from build123d import *

# Parameters (mm, degrees)
SKETCH1_R                  = 93.345
BASE_DEPTH                 = 4.7625
BASE_DEPTH_BACK            = 4.7625
BOTTOM_SUPPORT_HOLES_DEPTH = 10.525
BOTTOM_SUPPORT_GUIDE_DEPTH = 12.7
SKETCH6_R                  = 1.27
BOTTOM_BOLT_HOLE_DEPTH     = 12.7
TOP_SUPPORT_HOLES_DEPTH    = 4.7625
TOP_SUPPORT_GUIDE_DEPTH    = 12.7
SKETCH12_R                 = 1.27
TOP_BOLT_HOLE_DEPTH        = 12.7
BOTTOM_PATTERN_COUNT       = 4
CIRPATTERN3_COUNT          = 4


with BuildPart() as part:
    # Sketch1 → Base (new body, two sides)
    with BuildSketch(Plane(origin=(0, 0, 0), x_dir=(1, 0, 0), z_dir=(0, 1, 0))) as base_sk:
        Circle(SKETCH1_R)
    extrude(amount=BASE_DEPTH)
    extrude(base_sk.sketch, amount=-BASE_DEPTH_BACK)

    # Sketch2 → Bottom support holes (cut, through all)
    with BuildSketch(Plane(origin=(0, 4.7625, 0), x_dir=(1, 0, 0), z_dir=(0, 1, 0))):
        with BuildLine():
            Line((0, 88.9), (0, 83.82))
            ThreePointArc((0, 83.82), (-21.72026739, 80.956916842), (-41.956713931, 72.563258996))
            Line((-41.956713931, 72.563258996), (-44.39288973, 77.022602796))
            ThreePointArc((-44.39288973, 77.022602796), (-22.977169228, 85.879332172), (0, 88.9))
        make_face()
    bottom_support_holes = extrude(amount=-BOTTOM_SUPPORT_HOLES_DEPTH, mode=Mode.SUBTRACT)

    # Sketch3 → Bottom support guide (add)
    with BuildSketch(Plane(origin=(0, 4.7625, 0), x_dir=(1, 0, 0), z_dir=(0, 1, 0))):
        with BuildLine():
            Line((0, 83.82), (0, 76.2))
            ThreePointArc((0, 76.2), (-19.834896001, 73.573207764), (-38.302281481, 65.8739344))
            Line((-38.302281481, 65.8739344), (-41.956713931, 72.563258996))
            ThreePointArc((-41.956713931, 72.563258996), (-21.72026739, 80.956916842), (0, 83.82))
        make_face()
    bottom_support_guide = extrude(amount=BOTTOM_SUPPORT_GUIDE_DEPTH)

    # Sketch6 → Bottom bolt hole (cut, symmetric)
    with BuildSketch(Plane(origin=(-20.978356966, 0, -78.191629498), x_dir=(-0.965842482, 0, 0.25912989), z_dir=(-0.25912989, 0, -0.965842482))):
        with Locations((-0.00326739, 11.1125)):
            Circle(SKETCH6_R)
    bottom_bolt_hole = extrude(amount=BOTTOM_BOLT_HOLE_DEPTH, both=True, mode=Mode.SUBTRACT)

    # Sketch8 → Top support holes (cut)
    with BuildSketch(Plane(origin=(-31.122978549, 4.7625, 77.296707326), x_dir=(1, 0, 0), z_dir=(0, 1, 0))):
        with BuildLine():
            Line((-31.738814298, 140.158500173), (-28.14671185, 136.566397725))
            ThreePointArc((-28.14671185, 136.566397725), (-41.480754694, 119.183343848), (-49.854870889, 98.93880289))
            Line((-49.854870889, 98.93880289), (-54.730739557, 100.369398703))
            ThreePointArc((-54.730739557, 100.369398703), (-45.850191767, 121.775253295), (-31.738814298, 140.158500173))
        make_face()
    top_support_holes = extrude(amount=-TOP_SUPPORT_HOLES_DEPTH, mode=Mode.SUBTRACT)

    # Sketch10 → Top support guide (add)
    with BuildSketch(Plane(origin=(-31.122978549, 4.7625, 77.296707326), x_dir=(1, 0, 0), z_dir=(0, 1, 0))):
        with BuildLine():
            Line((-28.14671185, 136.566397725), (-22.758558177, 131.178244052))
            ThreePointArc((-22.758558177, 131.178244052), (-34.92652504, 115.295431983), (-42.540730139, 96.792810073))
            Line((-42.540730139, 96.792810073), (-49.854870889, 98.93880289))
            ThreePointArc((-49.854870889, 98.93880289), (-41.480754694, 119.183343848), (-28.14671185, 136.566397725))
        make_face()
    top_support_guide = extrude(amount=TOP_SUPPORT_GUIDE_DEPTH)

    # Sketch12 → Top bolt hole (cut, symmetric)
    with BuildSketch(Plane(origin=(-70.123769919, 0, -40.455892982), x_dir=(-0.499721266, 0, 0.866186271), z_dir=(-0.866186271, 0, -0.499721266))):
        with Locations((-0.00326739, 11.1125)):
            Circle(SKETCH12_R)
    top_bolt_hole = extrude(amount=TOP_BOLT_HOLE_DEPTH, both=True, mode=Mode.SUBTRACT)

    # Bottom pattern: Bottom support holes, Bottom support guide, Bottom bolt hole ×4 about axis
    bottom_pattern_axis = Axis((0, 0, 0), (0, 1, 0))
    for i in range(1, BOTTOM_PATTERN_COUNT):
        add(bottom_support_holes.rotate(bottom_pattern_axis, i * 360 / BOTTOM_PATTERN_COUNT), mode=Mode.SUBTRACT)
        add(bottom_support_guide.rotate(bottom_pattern_axis, i * 360 / BOTTOM_PATTERN_COUNT))
        add(bottom_bolt_hole.rotate(bottom_pattern_axis, i * 360 / BOTTOM_PATTERN_COUNT), mode=Mode.SUBTRACT)

    # CirPattern3: Top support holes, Top support guide, Top bolt hole ×4 about axis
    cirpattern3_axis = Axis((0, 0, 0), (0, 1, 0))
    for i in range(1, CIRPATTERN3_COUNT):
        add(top_support_holes.rotate(cirpattern3_axis, i * 360 / CIRPATTERN3_COUNT), mode=Mode.SUBTRACT)
        add(top_support_guide.rotate(cirpattern3_axis, i * 360 / CIRPATTERN3_COUNT))
        add(top_bolt_hole.rotate(cirpattern3_axis, i * 360 / CIRPATTERN3_COUNT), mode=Mode.SUBTRACT)


solid = part.part
Part model, mm, in its own coordinate system. A direction names the side the tool comes from. Give positions to 0.01 mm unless a question says otherwise; leave off trailing zeros. Loops run counter-clockwise (first coordinate to the right, second up) from the corner with the lowest first, then second, coordinate; pieces in that order, holes last.
(1) Band-saw the part on B-B (z = 57). Write the cut outline in (x, y), and give its area (3 significant figures).
Return value:
outline: (-73.92, -4.76) - (73.92, -4.76) - (73.92, 4.76) - (68.22, 4.76) - (68.22, 0) - (61.46, 0) - (61.46, 17.46) - (57, 17.46) - (57, 4.76) - (-50.57, 4.76) - (-50.57, 17.46) - (-57, 17.46) - (-57, 4.76) - (-73.92, 4.76) - close
area: 1,510 mm2
(2) Drill centre lines: line 1 along Z through (x, y) = (0.5, -1.75); line 2 along X through (y, z) = (2, 0.5); line 3 along Y through (x, z) = (-75, -47.5). Where is each one in solid material? Low to high.
Return value:
line 1: z = -93.34 to 83.82, 88.9 to 93.34
line 2: x = -93.34 to -88.9, -83.82 to 93.34
line 3: y = -4.76 to 0
(3) 3-axis set-ups, long thin cutter, end or side, ignore diameter. For faces 1 (the flat face through (0, 11, 80)), 2 (the flat face through (73, 0, 44)), 3 (the flat face through (-57, 11, -57)), 4 (the cylindrical face through (85.795, 0.067, -23.291)): which of +Z, -Z, +X, -X, +Y, -Y reach the whole face in a straight line?
Return value:
face 1: +Z, +Y
face 2: +Y
face 3: -Z, +Y
face 4: +Y, -Y
(4) Band-saw the part on A-A (z = -5.5). Write the cut outline in (x, y), and give its area (3 significant figures).
Return value:
outline: (-93.18, -4.76) - (83.64, -4.76) - (83.64, 17.46) - (76, 17.46) - (76, 4.76) - (-93.18, 4.76) - close; (88.73, -4.76) - (93.18, -4.76) - (93.18, 4.76) - (88.73, 4.76) - close
area: 1,820 mm2
(5) Pin check, flat tips, straight feed: pin 1 (10 mm diameter, centred on y = 7.5, z = -22, fed in from +X); pin 2 (4 mm diameter, centred on x = 78, y = 11, fed in from +Z); pin 3 (1.5 mm diameter, centred on x = 23, z = 13, fed in from +Y); pin 4 (8 mm diameter, centred on x = 70, z = 49.5, fed in from +Y). Stop position of each tip, or through.
Return value:
pin 1: stops at x = 91.63
pin 2: stops at z = 35.35
pin 3: stops at y = 4.76
pin 4: stops at y = 17.46
(6) Pull direction X, two halves, no side cores. Call faces 5 (the flat face through (22.347, 2.415, -83.382)), 6 (the flat face through (40.104, 11.024, 69.172)), 7 (the flat face through (68, 17.462, 41)): pulls with the +X half, pulls with the -X half, needs draft (parallel to the pull), parting line crosses it, or undercut.
Return value:
face 5: undercut
face 6: pulls with the +X half
face 7: needs draft
